Check sheet for the modelled part. Datum: model origin and axes. Units: mm. Face numbers are marked on the shaded views. A direction names the side the tool comes from. Round coordinates to 2 decimals unless told otherwise and drop trailing zeros. Order: outer loops, then holes, each group sorted by start corner. A loop starts at its lowest first (then second) coordinate and runs counter-clockwise, first axis right, second up. Notation, with made-up numbers: M 64.5,-23.5 L 89.5,-23.5 A22 ccw 89.5,1.5 Z; hole C -21.75,-24 d7. An arc over 180 degrees is marked long. One line per item, written item: value. Start each with the question number.
(1) Access from +Z, -Z, +X, -X, +Y, -Y to the whole of each face (thin tool, end or side, straight path). Record for the marked faces 1, 2, 3, 4 and 5.
(2) Cross-section at C-C, the plane x = 20. Enter the section's corners in (y, z), and give its area (3 significant figures).
(3) Cross-section at D-D, the plane y = 14. Enter the section's corners in (x, z), and give its area (3 significant figures).
(4) Cross-section at B-B, the plane y = 0. Enter the section's corners in (x, z).
(5) Thickness scan on L1, parallel to Y at x = -7, z = -4; L2, parallel to Y at x = -3, z = -4.5; L3, parallel to Y at x = 4, z = -1.75. Record the ranges inside material, lowest first.
(6) Cross-section at A-A, the plane z = -11.5. Enter the section's corners in (x, y).
(7) Depth check by flat-ended pin: pin 1 Ø5 at (x, z) = (9.5, -4) entering from +Y; pin 2 Ø4 at (x, y) = (16.5, 2) entering from +Z; pin 3 Ø4 at (y, z) = (-16.5, -9.5) entering from -X; pin 4 Ø13.5 at (x, y) = (2.5, -10) entering from +Z. Enter the tip coordinate at first touch or a pass-through.
(8) Release check for a two-part mould opening along X. For the marked faces 6, 7 and 8 record: released by +X, released by -X, zero draft, split by the parting line, or undercut.
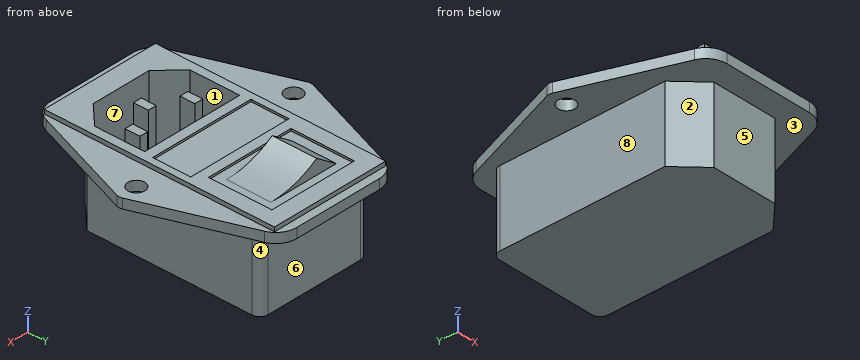
Autodesk Inventor part; units mm, degrees
ref_plane "YZ Plane" through (0, 0, 0) normal (1, 0, 0) x (0, 1, 0)
ref_plane "XZ Plane" through (0, 0, 0) normal (0, 1, 0) x (-1, 0, 0)
ref_plane "XY Plane" through (0, 0, 0) normal (0, 0, 1) x (1, 0, 0)
sketch "Sketch3" plane through (0, 0, 0) normal (0, 0, 1) x (1, 0, 0)
  line L0 (-13.75, 23.5) -> (13.75, 23.5)
  line L1 (13.75, 23.5) -> (13.75, -23.5)
  line L2 (13.75, -23.5) -> (-13.75, -23.5)
  line L3 (-13.75, -23.5) -> (-13.75, 23.5)
  line L4 (-13.75, 23.5) -> (13.75, -23.5) construction
  line L5 (13.75, 23.5) -> (-13.75, -23.5) construction
  point P0 (0, 0)
  dimension "d17" = 27.5
  dimension "d18" = 47
extrude "Extrusion1" add sketch "Sketch3" against normal blind 20
sketch "Sketch2" plane through (0, 0, 0) normal (0, 0, 1) x (1, 0, 0)
  line L0 (-24.5, 0) -> (24.5, 0) construction
  line L1 (0, 29.1) -> (0, -29.1) construction
  line L2 (-14, 29.1) -> (14, 29.1)
  line L3 (-14, 29.1) -> (-24.5, 0)
  line L4 (14, 29.1) -> (24.5, 0)
  line L5 (-14, -29.1) -> (14, -29.1)
  line L6 (-24.5, 0) -> (-14, -29.1)
  line L7 (24.5, 0) -> (14, -29.1)
  circle A0 centre (20, 0) radius 2
  circle A1 centre (-20, 0) radius 2
  point P0 (0, 0)
  point P1 (0, 0)
  dimension "d12" = 49
  dimension "d13" = 58.2
  dimension "d14" = 28
  dimension "d15" = 4
  dimension "d16" = 40
extrude "Extrusion2" add sketch "Sketch2" against normal blind 2.3
sketch "Sketch1" plane through (0, 0, 0) normal (0, 0, 1) x (1, 0, 0)
  line L0 (-14.15, 27.2) -> (14.15, 27.2)
  line L1 (14.15, 27.2) -> (14.15, -27.2)
  line L2 (14.15, -27.2) -> (-14.15, -27.2)
  line L3 (-14.15, -27.2) -> (-14.15, 27.2)
  line L4 (-14.15, 27.2) -> (14.15, -27.2) construction
  line L5 (14.15, 27.2) -> (-14.15, -27.2) construction
  line L6 (-10.5, 23.2) -> (10.5, 23.2)
  line L7 (10.5, 23.2) -> (10.5, 8.2)
  line L8 (10.5, 8.2) -> (-10.5, 8.2)
  line L9 (-10.5, 8.2) -> (-10.5, 23.2)
  line L10 (-10.5, 23.2) -> (10.5, 8.2) construction
  line L11 (10.5, 23.2) -> (-10.5, 8.2) construction
  line L12 (0, 15.7) -> (0, 0) construction
  line L13 (-12.1, -5.4) -> (12.1, -5.4)
  line L14 (12.1, -5.4) -> (12.1, -22.2)
  line L15 (12.1, -22.2) -> (-12.1, -22.2)
  line L16 (-12.1, -22.2) -> (-12.1, -5.4)
  line L17 (-12.1, -5.4) -> (12.1, -22.2) construction
  line L18 (12.1, -5.4) -> (-12.1, -22.2) construction
  line L19 (0, 0) -> (0, -13.8) construction
  line L20 (-8.3, 20.95) -> (8.3, 20.95)
  line L21 (8.3, 20.95) -> (8.3, 10.45)
  line L22 (8.3, 10.45) -> (-8.3, 10.45)
  line L23 (-8.3, 10.45) -> (-8.3, 20.95)
  line L24 (-8.3, 20.95) -> (8.3, 10.45) construction
  line L25 (8.3, 20.95) -> (-8.3, 10.45) construction
  line L26 (-12.5, 5.8689) -> (12.5, 5.8689)
  line L27 (12.5, 5.8689) -> (12.5, -3.1311)
  line L28 (12.5, -3.1311) -> (-12.5, -3.1311)
  line L29 (-12.5, -3.1311) -> (-12.5, 5.8689)
  line L30 (-12.5, 5.8689) -> (12.5, -3.1311) construction
  line L31 (12.5, 5.8689) -> (-12.5, -3.1311) construction
  point P0 (0, 1.3689)
  dimension "d0" = 28.3
  dimension "d1" = 54.4
  dimension "d2" = 21
  dimension "d3" = 15
  dimension "d4" = 4
  dimension "d5" = 24.2
  dimension "d6" = 16.8
  dimension "d7" = 5
  dimension "d8" = 16.6
  dimension "d9" = 10.5
  dimension "d10" = 25
  dimension "d11" = 9
extrude "Extrusion3" add sketch "Sketch1" along normal blind 1 contours L0 L1 L2 L3
extrude "Extrusion4" add sketch "Sketch1" along normal blind 0.5 contours L6 L7 L8 L9 | L26 L27 L28 L29
extrude "Extrusion5" add sketch "Sketch1" along normal blind 4 contours L20 L21 L22 L23
sketch "Sketch4" plane through (-8.3, 20.95, 0.5) normal (0, 1, 0) x (1, 0, 0)
  line L0 (0, -3.5) -> (16.6, -3.5)
  line L1 (0, 0) -> (0, -3.5)
  line L2 (16.6, 0) -> (16.6, -3.5)
  line L3 (0, 0) -> (5, -3.5)
  arc A0 (16.6, 0) -> (5, -3.5) centre (16.6082, -21) ccw
  point P0 (8.3, 0.5)
  dimension "d29" = 5
  dimension "d30" = 21
extrude "Extrusion6" cut sketch "Sketch4" against normal up to surface (10.5 mm away)
extrude "Extrusion7" cut sketch "Sketch1" against normal blind 19 contours L13 L14 L15 L16
sketch "Sketch5" plane through (0, 0, 0) normal (0, 0, 1) x (1, 0, 0)
  line L0 (-1, -14.8319) -> (1, -14.8319)
  line L1 (1, -14.8319) -> (1, -18.3319)
  line L2 (1, -18.3319) -> (-1, -18.3319)
  line L3 (-1, -18.3319) -> (-1, -14.8319)
  line L4 (-8, -10.3319) -> (-6, -10.3319)
  line L5 (-6, -10.3319) -> (-6, -13.8319)
  line L6 (-6, -13.8319) -> (-8, -13.8319)
  line L7 (-8, -13.8319) -> (-8, -10.3319)
  line L8 (6, -10.3319) -> (8, -10.3319)
  line L9 (8, -10.3319) -> (8, -13.8319)
  line L10 (8, -13.8319) -> (6, -13.8319)
  line L11 (6, -13.8319) -> (6, -10.3319)
  line L12 (-8, -12.0819) -> (8, -12.0819) construction
  line L13 (0, -14.8319) -> (0, -12.0819) construction
  point P0 (0, 0)
  dimension "d35" = 2
  dimension "d36" = 3.5
  dimension "d42" = 16
  dimension "d43" = 8
extrude "Extrusion8" add sketch "Sketch5" against normal up to next
fillet "Fillet1" radius 2 4 edges at (13.75, 23.5, -11.15) (-13.75, 23.5, -11.15) (24.5, 0, -1.15) (-24.5, 0, -1.15)
fillet "Fillet2" radius 5 4 edges at (14, 29.1, -1.15) (-14, 29.1, -1.15) (14, -29.1, -1.15) (-14, -29.1, -1.15)
chamfer "Chamfer1" distance 5 angle 45 2 edges at (12.1, -22.2, -9) (-12.1, -22.2, -9)
chamfer "Chamfer2" distance 6 angle 45 2 edges at (-13.75, -23.5, -11.15) (13.75, -23.5, -11.15)
properties part number "power-port" material "UHMW, Black"
Values found:
1. face 1: +Z
1. face 2: -Z, -X, -Y
1. face 3: -Z
1. face 4: -Z, +X, +Y
1. face 5: -Z, +X, -X, -Y
2. outline: M -12.47,-2.3 L -2,-2.3 L -2,0 L -12.47,0 Z; M 2,-2.3 L 12.47,-2.3 L 12.47,0 L 2,0 Z
2. area: 48.2 mm^2
3. outline: M -19.45,-2.3 L -13.75,-2.3 L -13.75,-20 L 13.75,-20 L 13.75,-2.3 L 19.45,-2.3 L 19.45,0 L 14.15,0 L 14.15,1 L 10.5,1 L 10.5,0.5 L 8.3,0.5 A21 cw -3.3,4 L -8.3,0.5 L -10.5,0.5 L -10.5,1 L -14.15,1 L -14.15,0 L -19.45,0 Z
3. area: 616 mm^2
4. outline: M -24.37,-2.3 L -22,-2.3 L -22,0 L -24.37,0 Z; M -18,-2.3 L -13.75,-2.3 L -13.75,-20 L 13.75,-20 L 13.75,-2.3 L 18,-2.3 L 18,0 L 14.15,0 L 14.15,1 L 12.5,1 L 12.5,0.5 L -12.5,0.5 L -12.5,1 L -14.15,1 L -14.15,0 L -18,0 Z; M 22,-2.3 L 24.37,-2.3 L 24.37,0 L 22,0 Z
5. L1: -23.5 to -22.2, -13.83 to -10.33, -5.4 to 23.5
5. L2: -23.5 to -22.2, -5.4 to 23.5
5. L3: -29.1 to -22.2, -5.4 to 29.1
6. outline: M -13.75,-17.5 L -7.75,-23.5 L 7.75,-23.5 L 13.75,-17.5 L 13.75,21.5 A2 ccw 11.75,23.5 L -11.75,23.5 A2 ccw -13.75,21.5 Z; M -8,-13.83 L -6,-13.83 L -6,-10.33 L -8,-10.33 Z; M -1,-18.33 L 1,-18.33 L 1,-14.83 L -1,-14.83 Z; M 6,-13.83 L 8,-13.83 L 8,-10.33 L 6,-10.33 Z; hole M -12.1,-17.2 L -7.1,-22.2 L 7.1,-22.2 L 12.1,-17.2 L 12.1,-5.4 L -12.1,-5.4 Z
7. pin 1: y = 29.1
7. pin 2: z = 0
7. pin 3: x = -13.75
7. pin 4: z = 1
8. face 6: zero draft
8. face 7: undercut
8. face 8: released by -X
